Check sheet for the drawn part. Datum: minimum x, y, z corner. Units: mm. A direction names the side the tool comes from. Coordinates: 2 decimals unless noted, no trailing zeros. Order: outer loops, then holes, each group sorted by start corner. A loop starts at its lowest first (then second) coordinate and runs counter-clockwise, first axis right, second up. Notation, with made-up numbers: (87, -40) - (108, -40) arc R14 cw to (108, -29) - close; hole circle Ø9 at (-40, 83.5). An arc over 180 degrees is marked (long way). Put each result on its own line as item: value.
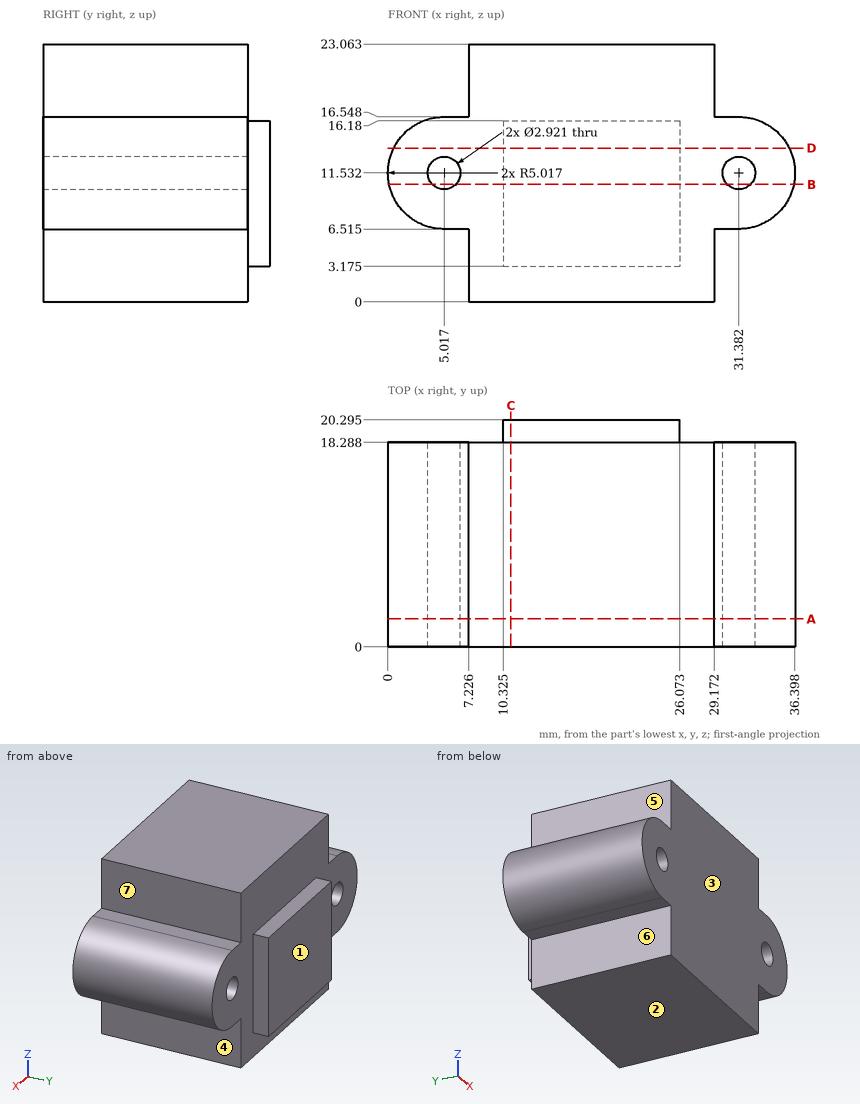
Q1. Draft check along Y on the marked faces 1, 2 and 3. Enter one of: pulls with the +Y half, pulls with the -Y half, needs draft (parallel to the pull), parting line crosses it, or undercut.
Answer block:
face 1: pulls with the +Y half
face 2: needs draft
face 3: pulls with the -Y half
Q2. Depth check by flat-ended pin: pin 1 Ø1.5 at (y, z) = (16, 19.5) entering from +X; pin 2 Ø3.5 at (y, z) = (5.5, 3.5) entering from -X; pin 3 Ø0.6 at (y, z) = (19, 8.5) entering from +X. Enter the tip coordinate at first touch or a pass-through.
Answer block:
pin 1: stops at x = 29.17
pin 2: stops at x = 7.23
pin 3: stops at x = 26.07
Q3. Section check A-A on y = 2.5. Record the boundary of the cut face in (x, z) (1 decimal), then the cut area to 3 significant figures.
Answer block:
outline: (5, 6.5) - (7.2, 6.5) - (7.2, 0) - (29.2, 0) - (29.2, 6.5) - (31.4, 6.5) arc R5 ccw to (31.4, 16.5) - (29.2, 16.5) - (29.2, 23.1) - (7.2, 23.1) - (7.2, 16.5) - (5, 16.5) arc R5 ccw to start; hole circle Ø2.9 at (5, 11.5); hole circle Ø2.9 at (31.4, 11.5)
area: 616 mm^2
Q4. Thickness scan on L1, parallel to X at y = 2.75, z = 1; L2, parallel to Y at x = 32.5, z = 10; L3, parallel to Z at x = 2, y = 3.5 (1 decimal). Record the ranges inside material, lowest first. Write a range as [from, to].
Answer block:
L1: x = [7.23, 29.17]
L2: y = [0, 18.29]
L3: z = [7.5, 15.5]
Q5. Section check B-B on z = 10.5. State how many separate pieces and enclosed holes the cut face has, then the cut area to 3 significant figures.
Answer block:
separate pieces: 3
enclosed holes: 0
area: 618 mm^2
Q6. Section check C-C on x = 11. Record the boundary of the cut face in (y, z) (1 decimal).
Answer block:
outline: (0, 0) - (18.3, 0) - (18.3, 3.2) - (20.3, 3.2) - (20.3, 16.2) - (18.3, 16.2) - (18.3, 23.1) - (0, 23.1) - close
Q7. Access from +Z, -Z, +X, -X, +Y, -Y to the whole of each face (thin tool, end or side, straight path). Record for the marked faces 4, 5, 6 and 7.
Answer block:
face 4: -Z, +X, +Y, -Y
face 5: +Z, -X, +Y, -Y
face 6: -Z, -X, +Y, -Y
face 7: +Z, +X, +Y, -Y
Q8. Section check D-D on z = 13.75. Record the boundary of the cut face in (x, y) (1 decimal).
Answer block:
outline: (0.5, 0) - (35.9, 0) - (35.9, 18.3) - (26.1, 18.3) - (26.1, 20.3) - (10.3, 20.3) - (10.3, 18.3) - (0.5, 18.3) - close
